Source: CAD feature listing. Evaluate the final solid. Frame: model axes, mm. A direction names the side the tool comes from. Coordinates: 2 decimals unless noted, no trailing zeros. Order: outer loops, then holes, each group sorted by start corner. A loop starts at its lowest first (then second) coordinate and runs counter-clockwise, first axis right, second up. Notation, with made-up numbers: (79.5, 10.5) -> (117.5, 10.5) arc R14 cw to (117.5, 24.5) -> close; hole circle Ø1 at (-37.5, 35). An arc over 180 degrees is marked (long way). Write each question's results on one line, items separated by ' | '. Start each with the question number.
from build123d import *

# Parameters (mm, degrees)
SKETCH2_W           = 197.612
SKETCH2_H           = 109.982
BOSS_EXTRUDE1_DEPTH = 12.7
SKETCH3_W           = 19.05
SKETCH3_H           = 25.4
BOSS_EXTRUDE2_DEPTH = 15.5575


with BuildPart() as part:
    # Sketch1 → Revolve1 (revolve)
    with BuildSketch(Plane.XY):
        with BuildLine():
            Line((103.6447, -10.668), (103.6447, -15.748))
            ThreePointArc((103.6447, -15.748), (105.9307, -18.034), (103.6447, -20.32))
            Line((103.6447, -20.32), (103.6447, -26.2255))
            Line((103.6447, -26.2255), (97.7392, -26.2255))
            ThreePointArc((97.7392, -26.2255), (95.4532, -28.5115), (93.1672, -26.2255))
            Line((93.1672, -26.2255), (88.0872, -26.2255))
            Line((88.0872, -26.2255), (88.0872, -38.9255))
            Line((88.0872, -38.9255), (116.3447, -38.9255))
            Line((116.3447, -38.9255), (116.3447, -10.668))
            Line((116.3447, -10.668), (103.6447, -10.668))
        make_face()
    revolve(axis=Axis((0, 0, 0), (0, -1, 0)))

    # Sketch2 → Boss-Extrude1 (add)
    with BuildSketch(Plane.XZ.offset(38.9255)):
        Rectangle(SKETCH2_W, SKETCH2_H)
    extrude(amount=BOSS_EXTRUDE1_DEPTH)

    # Sketch3 → Boss-Extrude2 (add)
    with BuildSketch(Plane(origin=(0, -10.668, 0), x_dir=(1, 0, 0), z_dir=(0, 1, 0))):
        with Locations((123.825, 0)):
            Rectangle(SKETCH3_W, SKETCH3_H)
        with Locations((-123.825, 0)):
            Rectangle(SKETCH3_W, SKETCH3_H)
    extrude(amount=-BOSS_EXTRUDE2_DEPTH)


solid = part.part
(1) First-contact query: P1, Ø8, axis at y = -44.5, z = -19, coming from the -X side; P2, Ø2, axis at y = -20, z = -20.5, coming from the -X side; P3, Ø8, axis at x = 29, y = -43.5, coming from the +Z side. Flat tips, straight axial feed; report the tip coordinate or a pass-through.
(2) Section B-B on z = 0. Return the cut outline in (x, y), then the cut area to 3 significant figures.
(3) Section A-A on x = 0. Return the cut outline in (y, z), then the cut area to 3 significant figures.
(4) Reachability of faces 1 (the flat face through (76, -26.226, 62)), 2 (the flat face through (98.806, -45, -1)), 3 (the flat face through (-125, -18, -12.7)) from +Z, -Z, +X, -X, +Y, -Y: full face, straight path, thin tool, end or side. Return the list, or none.
(5) Section D-D on x = 46.5. Count the separate pieces of the cut face and the enclosed holes in it, then the cut area to 3 significant figures.
(6) Section C-C on y = -48. Return the cut outline in (x, z).
(7) Line query: L1, parallel to Z at x = 0, y = -12.2; L2, parallel to X at y = -32.75, z = 0. Output: solid intervals per line, ascending.
Results list:
1) P1: stops at x = -98.81 | P2: stops at x = -114.7 | P3: stops at z = 54.99
2) outline: (-133.35, -26.23) -> (-116.34, -26.23) -> (-116.34, -38.93) -> (-98.81, -38.93) -> (-98.81, -51.63) -> (98.81, -51.63) -> (98.81, -38.93) -> (116.34, -38.93) -> (116.34, -26.23) -> (133.35, -26.23) -> (133.35, -10.67) -> (103.64, -10.67) -> (103.64, -15.75) arc R2.29 cw to (103.64, -20.32) -> (103.64, -26.23) -> (97.74, -26.23) arc R2.29 cw to (93.17, -26.23) -> (88.09, -26.23) -> (88.09, -38.93) -> (-88.09, -38.93) -> (-88.09, -26.23) -> (-93.17, -26.23) arc R2.29 cw to (-97.74, -26.23) -> (-103.64, -26.23) -> (-103.64, -20.32) arc R2.29 cw to (-103.64, -15.75) -> (-103.64, -10.67) -> (-133.35, -10.67) -> close | area: 4,120 mm²
3) outline: (-51.63, -54.99) -> (-38.93, -54.99) -> (-38.93, 54.99) -> (-51.63, 54.99) -> close; (-38.93, -116.34) -> (-10.67, -116.34) -> (-10.67, -103.64) -> (-15.75, -103.64) arc R2.29 cw to (-20.32, -103.64) -> (-26.23, -103.64) -> (-26.23, -97.74) arc R2.29 cw to (-26.23, -93.17) -> (-26.23, -88.09) -> (-38.93, -88.09) -> close; (-38.93, 88.09) -> (-26.23, 88.09) -> (-26.23, 93.17) arc R2.29 cw to (-26.23, 97.74) -> (-26.23, 103.64) -> (-20.32, 103.64) arc R2.29 cw to (-15.75, 103.64) -> (-10.67, 103.64) -> (-10.67, 116.34) -> (-38.93, 116.34) -> close | area: 2,480 mm²
4) face 1: +Y | face 2: +Z, -Z, +X, -Y | face 3: -Z, -X, +Y, -Y
5) separate pieces: 3 | enclosed holes: 0 | area: 2,600 mm²
6) outline: (-98.81, -54.99) -> (98.81, -54.99) -> (98.81, 54.99) -> (-98.81, 54.99) -> close
7) L1: z = -116.34 to -103.64, 103.64 to 116.34 | L2: x = -116.34 to -88.09, 88.09 to 116.34
